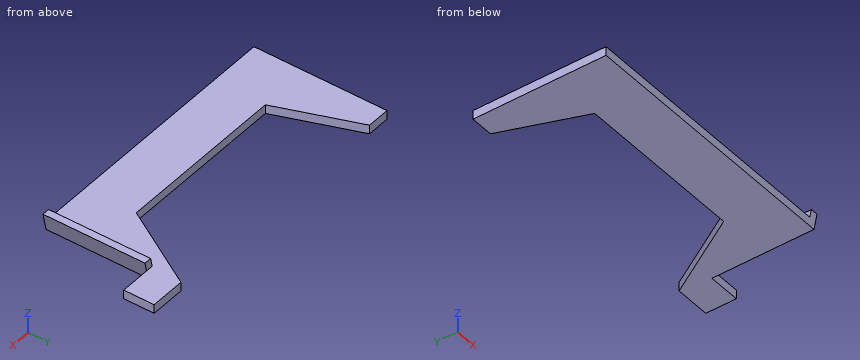
from build123d import *

# Parameters (mm, degrees)
BOSS_EXTRUDE1_DEPTH = 2
BOSS_EXTRUDE2_DEPTH = 46


with BuildPart() as part:
    # Sketch1 → Boss-Extrude1 (new, symmetric)
    with BuildSketch(Plane.XY):
        Polygon((-60.75, -30), (-60.75, 30), (-50.352877454, 30), (-36.945370579, -6.855179418), (39.897088693, -6.855179418), (61.606830496, 29.73214036), (77.549740604, 29.73214036), (77.549740604, 16), (63.049740604, 16), (63.049740604, -30), align=None)
    extrude(amount=BOSS_EXTRUDE1_DEPTH, both=True)

    # Sketch2 → Boss-Extrude2 (add)
    with BuildSketch(Plane.XZ.offset(30)):
        Polygon((63.049740604, -2), (64.873027277, 6.219294114), (61.530350142, 6.219294114), (60.59438379, 2), align=None)
    extrude(amount=-BOSS_EXTRUDE2_DEPTH)


solid = part.part
Geometry: final body of the model. Coordinates: model frame, mm. Give positions to 0.01 mm unless a question says otherwise; leave off trailing zeros. Write each loop counter-clockwise with the first axis right and the second up, starting at its lowest first coordinate (ties: lowest second). Pieces come first, ordered by that corner, then holes.
(1) First-contact query: P1, Ø1, axis at x = 49, y = -19.5, coming from the +Z side; P2, Ø3.5, axis at x = 63, z = 5, coming from the +Y side; P3, Ø2, axis at y = 21.5, z = 4.5, coming from the +X side; P4, Ø2, axis at y = 5.5, z = 1, coming from the +X side. Flat tips, straight axial feed; report the tip coordinate or a pass-through.
(2) Cut plane B-B, the plane y = -13.5. Return loops of the section in (x, z), then the cut area to 3 significant figures.
(3) Cut plane A-A, the plane y = 18. Return loops of the section in (x, z), then the cut area to 3 significant figures.
(4) Ray query, line 1 (Y direction, x = 15.5, z = 0.75); line 2 (Z direction, x = 52.5, y = -17.5); line 3 (X direction, y = 9.5, z = -1.25). Return the intervals inside material, ascending.
(5) Cut plane C-C, the plane y = 1. Return loops of the section in (x, z).
(6) Cut plane D-D, the plane x = 2. Return loops of the section in (y, z), then the cut area to 3 significant figures.
Values follow:
1. P1: stops at z = 2
1. P2: stops at y = 16
1. P3: passes through
1. P4: stops at x = 63.94
2. outline: (-60.75, -2) - (63.05, -2) - (64.87, 6.22) - (61.53, 6.22) - (60.59, 2) - (-60.75, 2) - close
2. area: 511 mm2
3. outline: (-60.75, -2) - (-45.99, -2) - (-45.99, 2) - (-60.75, 2) - close; (54.65, -2) - (77.55, -2) - (77.55, 2) - (54.65, 2) - close
3. area: 151 mm2
4. line 1: y = -30 to -6.86
4. line 2: z = -2 to 2
4. line 3: x = -60.75 to -42.9, 49.6 to 63.22
5. outline: (-60.75, -2) - (-39.8, -2) - (-39.8, 2) - (-60.75, 2) - close; (44.56, -2) - (63.05, -2) - (64.87, 6.22) - (61.53, 6.22) - (60.59, 2) - (44.56, 2) - close
6. outline: (-30, -2) - (-6.86, -2) - (-6.86, 2) - (-30, 2) - close
6. area: 92.6 mm2
